Autodesk Fusion 360 part; units mm, degrees
sketch "Sketch1" plane through (0, 0, 0) normal (0, 0, 1) x (1, 0, 0)
  line L0 (-39.1988, 50) -> (50.8012, 50)
  line L1 (50.8012, 50) -> (50.8012, -50)
  line L2 (50.8012, -50) -> (-39.1988, -50)
  line L3 (-39.1988, -50) -> (-39.1988, 50)
  line L4 (-43.1988, -60) -> (54.8012, -60)
  line L5 (60.8012, -54) -> (60.8012, 54)
  line L6 (54.8012, 60) -> (-43.1988, 60)
  line L7 (-49.1988, 54) -> (-49.1988, -54)
  circle A0 centre (9.8012, -55) radius 3.1
  circle A1 centre (54.8012, -54) radius 3.1
  circle A2 centre (-43.1988, -54) radius 3.1
  circle A3 centre (55.8012, 0) radius 3.1
  circle A4 centre (54.8012, 54) radius 3.1
  circle A5 centre (-44.1988, 0) radius 3.1
  circle A6 centre (-43.1988, 54) radius 3.1
  circle A7 centre (5.8012, 55) radius 3.1
  arc A8 (-49.1988, -54) -> (-43.1988, -60) centre (-43.1988, -54) ccw
  arc A9 (54.8012, -60) -> (60.8012, -54) centre (54.8012, -54) ccw
  arc A10 (60.8012, 54) -> (54.8012, 60) centre (54.8012, 54) ccw
  arc A11 (-43.1988, 60) -> (-49.1988, 54) centre (-43.1988, 54) ccw
  dimension "d1" = 90
  dimension "d5" = 10
  dimension "d6" = 10
  dimension "d7" = 6.2
  dimension "d8" = 6.2
  dimension "d9" = 6.2
  dimension "d10" = 6
  dimension "d11" = 6
  dimension "d12" = 6
  dimension "d13" = 6
  dimension "d14" = 59
  dimension "d15" = 6.2
  dimension "d16" = 6.2
  dimension "d17" = 6
  dimension "d18" = 6
  dimension "d19" = 60
  dimension "d20" = 6.2
  dimension "d21" = 5
  dimension "d22" = 5
  dimension "d23" = 5
  dimension "d24" = 6.2
  dimension "d25" = 6
  dimension "d26" = 6
  dimension "d27" = 60
  dimension "d28" = 6.2
  dimension "d29" = 5
  dimension "d30" = 55
  dimension "d31" = 6
  dimension "d32" = 6
  dimension "d33" = 6
  dimension "d34" = 6
extrude "Extrude1" add sketch "Sketch1" along normal blind 55
extrude "Extrude2" add sketch "Sketch1" along normal blind 3.2 contours L0 L1 L2 L3
extrude "Extrude3" add sketch "Sketch1" along normal blind 51.85 contours A0 | A1 | A2 | A3 | A4 | A5 | A6 | A7
Build history of the part. All positions in model axes, mm. A direction names the side the tool comes from. Round coordinates to 2 decimals unless told otherwise and drop trailing zeros. Order: outer loops, then holes, each group sorted by start corner. A loop starts at its lowest first (then second) coordinate and runs counter-clockwise, first axis right, second up. Notation, with made-up numbers: (-39, -7) - (-22, -7) arc R32 cw to (-22, 21) - close; hole circle Ø11 at (63, 61). An arc over 180 degrees is marked (long way). Use a Markdown table: item, result.
1) Flat gauge pins, fed straight in: pin 1 Ø5 at (x, y) = (54.8, 54) entering from -Z; pin 2 Ø6 at (x, y) = (10, -39) entering from +Z; pin 3 Ø3 at (x, y) = (6, 54.5) entering from +Z. Where does each tip first touch, or does it go through?
Recorded:
| item | result |
|---|---|
| pin 1 | stops at z = 0 |
| pin 2 | stops at z = 3.2 |
| pin 3 | stops at z = 51.85 |
2) Saw through at C-C on y = -43. Write the cut outline in (x, z), and give its area (3 significant figures).
Recorded:
| item | result |
|---|---|
| outline | (-49.2, 0) - (60.8, 0) - (60.8, 55) - (50.8, 55) - (50.8, 3.2) - (-39.2, 3.2) - (-39.2, 55) - (-49.2, 55) - close |
| area | 1,390 mm² |
3) Pull direction Y, two halves, no side cores. Call faces 3 (the face through (58.997, 58.289, 27.115)), 4 (the face through (6, 55, 51.85)), 5 (the face through (60.801, -1, 27)): pulls with the +Y half, pulls with the -Y half, needs draft (parallel to the pull), parting line crosses it, or undercut.
Recorded:
| item | result |
|---|---|
| face 3 | pulls with the +Y half |
| face 4 | undercut |
| face 5 | needs draft |
4) Saw through at A-A on z = 34. Write the cut outline in (x, y), and give its area (3 significant figures).
Recorded:
| item | result |
|---|---|
| outline | (-49.2, -54) arc R6 ccw to (-43.2, -60) - (54.8, -60) arc R6 ccw to (60.8, -54) - (60.8, 54) arc R6 ccw to (54.8, 60) - (-43.2, 60) arc R6 ccw to (-49.2, 54) - close; hole (-39.2, -50) - (50.8, -50) - (50.8, 50) - (-39.2, 50) - close |
| area | 4,170 mm² |
5) Saw through at B-B on x = -23. Write the cut outline in (y, z), and give its area (3 significant figures).
Recorded:
| item | result |
|---|---|
| outline | (-60, 0) - (60, 0) - (60, 55) - (50, 55) - (50, 3.2) - (-50, 3.2) - (-50, 55) - (-60, 55) - close |
| area | 1,420 mm² |
6) Tool access for faces 1 (the face through (-47.488, 58.196, 27.115)), 2 (the face through (50.801, 1, 29)): list every direction of +Z, -Z, +X, -X, +Y, -Y with a clear straight run to the whole face (end or side of a thin tool).
Recorded:
| item | result |
|---|---|
| face 1 | +Z, -Z, -X, +Y |
| face 2 | +Z |
7) Wall check: L1, parallel to Y at x = 33.5, z = 8.5; L2, parallel to X at y = -3, z = 9; L3, parallel to Z at x = -7, y = 36. Give the ranges that are in metal, low to high.
Recorded:
| item | result |
|---|---|
| L1 | y = -60 to -50, 50 to 60 |
| L2 | x = -49.2 to -39.2, 50.8 to 60.8 |
| L3 | z = 0 to 3.2 |
